Answer from the drawing. Dimensions are ordinates in mm from the lowest x, y and z of the part. Coordinates: 2 decimals unless noted, no trailing zeros. Write each loop counter-clockwise with the first axis right and the second up, starting at its lowest first coordinate (ties: lowest second). Pieces come first, ordered by that corner, then holes. Notation, with made-up numbers: (52.25, 12) - (99.25, 12) arc R29 ccw to (99.25, 41) - close; hole circle Ø1 at (19.25, 44). An arc over 180 degrees is marked (long way). Answer as a JSON object with one key per item and string values. Group by question number.
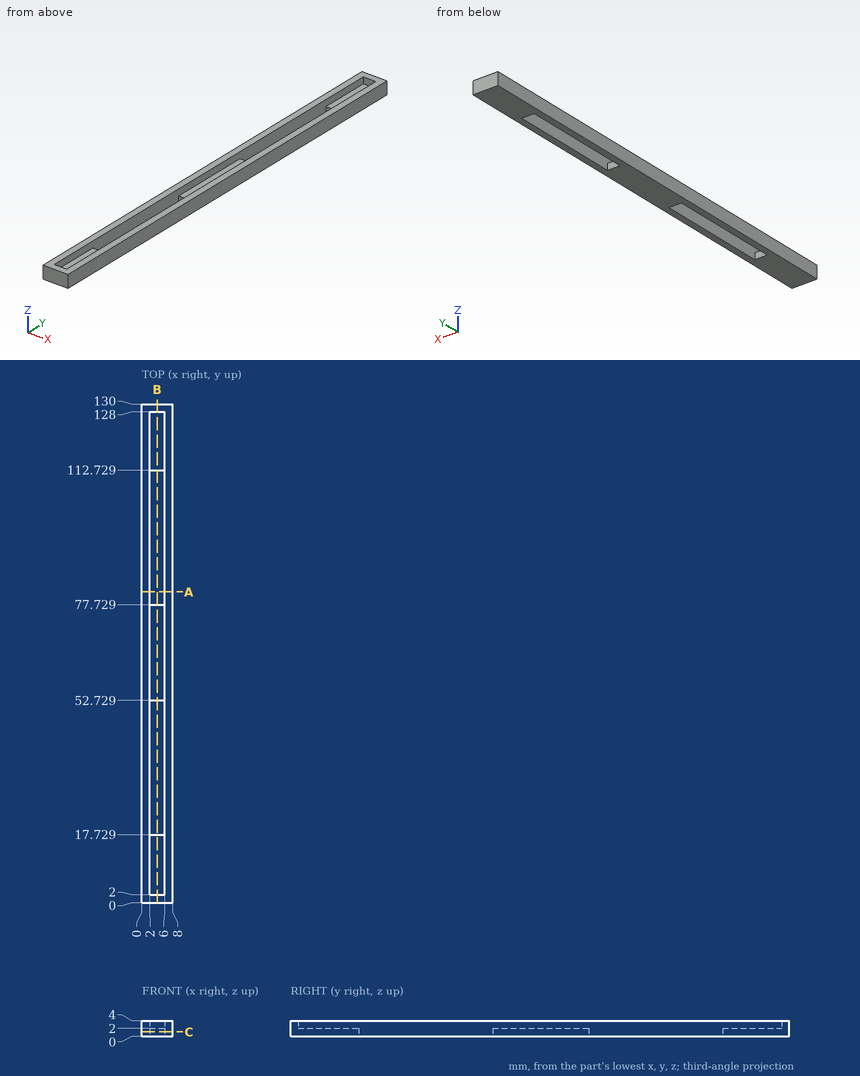
Q1. Flat-ended cylindrical pins translate along their axes: pin 1 Ø1 at (x, z) = (4.5, 0.5) entering from -Y; pin 2 Ø2 at (x, y) = (4, 60.5) entering from +Z. Find the tip coordinate at first contact, or state that the pin passes through.
Q2. Section C-C on z = 1.1 is taken. Determine the outline of the cut face in (x, y), plus the area to 3 significant figures.
Q3. Section A-A on y = 81 is taken. Determine the outline of the cut face in (x, z).
Q4. Section B-B on x = 4 is taken. Determine the outline of the cut face in (y, z), plus the area to 3 significant figures.
Q5. Consider L1, parallel to Y at x = 4.5, z = 1.55; L2, parallel to X at y = 101.5, z = 2.45; L3, parallel to Y at x = 4.5, z = 2.5. Determine where each line is inside the solid, lowest interval first. Write a range as from..to.
Numbers:
{
 "1": {"pin 1": "stops at y = 0", "pin 2": "stops at z = 2"},
 "2": {"outline": "(0, 0) - (8, 0) - (8, 130) - (0, 130) - close; hole (2, 17.73) - (6, 17.73) - (6, 52.73) - (2, 52.73) - close; hole (2, 77.73) - (6, 77.73) - (6, 112.73) - (2, 112.73) - close", "area": "760 mm²"},
 "3": {"outline": "(0, 0) - (2, 0) - (2, 4) - (0, 4) - close; (6, 0) - (8, 0) - (8, 4) - (6, 4) - close"},
 "4": {"outline": "(0, 0) - (17.73, 0) - (17.73, 2) - (2, 2) - (2, 4) - (0, 4) - close; (52.73, 0) - (77.73, 0) - (77.73, 2) - (52.73, 2) - close; (112.73, 0) - (130, 0) - (130, 4) - (128, 4) - (128, 2) - (112.73, 2) - close", "area": "128 mm²"},
 "5": {"L1": "y = 0..17.73, 52.73..77.73, 112.73..130", "L2": "x = 0..2, 6..8", "L3": "y = 0..2, 128..130"}
}
